CAD build for the part. Positions are in the model's coordinates, mm. A direction names the side the tool comes from. Round coordinates to 2 decimals unless told otherwise and drop trailing zeros. Loops run counter-clockwise (first coordinate to the right, second up) from the corner with the lowest first, then second, coordinate; pieces in that order, holes last. Notation, with made-up numbers: M -2.75,16.25 L 25.25,16.25 A10 cw 25.25,22.25 Z; hole C 11,59 d2. An arc over 180 degrees is marked long. One line per item, written item: value. Start each with the question number.
from build123d import *

# Parameters (mm, degrees)
AUFSATZ_LINEAR_AUSTRAGEN1_DEPTH = 8
DURCHGANGSLOCH_F_R_M5_D         = 5.5
DURCHGANGSLOCH_F_R_M4_D         = 4.5


with BuildPart() as part:
    # Skizze1 → Aufsatz-Linear austragen1 (new body)
    with BuildSketch(Plane.XY):
        with BuildLine():
            Line((4.5, -24.047375097), (-4.5, -24.047375097))
            ThreePointArc((-4.5, -24.047375097), (-6.621320344, -24.926054753), (-7.5, -27.047375097))
            Line((-7.5, -27.047375097), (-7.5, -28.047375097))
            Line((-7.5, -28.047375097), (-10.646349149, -28.047375097))
            ThreePointArc((-10.646349149, -28.047375097), (-15, -25.980762114), (-18.966564769, -23.243696368))
            Line((-18.966564769, -23.243696368), (-20.539739343, -20.518878077))
            Line((-20.539739343, -20.518878077), (-19.673713939, -20.018878077))
            ThreePointArc((-19.673713939, -20.018878077), (-18.27593646, -18.197259001), (-18.575637728, -15.920801865))
            Line((-18.575637728, -15.920801865), (-23.075637728, -8.126573231))
            ThreePointArc((-23.075637728, -8.126573231), (-24.897256804, -6.728795752), (-27.173713939, -7.02849702))
            Line((-27.173713939, -7.02849702), (-28.039739343, -7.52849702))
            Line((-28.039739343, -7.52849702), (-29.612913917, -4.803678728))
            ThreePointArc((-29.612913917, -4.803678728), (-28.775894551, 8.482210373), (-22.272727273, 20.097900881))
            ThreePointArc((-22.272727273, 20.097900881), (-21.699837667, 21.031080126), (-21.5, 22.107690969))
            Line((-21.5, 22.107690969), (-21.5, 38.107690969))
            Line((-21.5, 38.107690969), (-16.5, 40.107690969))
            Line((-16.5, 40.107690969), (-1.5, 40.107690969))
            Line((-1.5, 40.107690969), (-1.5, 8.9))
            Line((-1.5, 8.9), (-5.75, 8.9))
            ThreePointArc((-5.75, 8.9), (-10.871320344, 11.021320344), (-8.75, 5.9))
            Line((-8.75, 5.9), (-8.75, -5.459334644))
            ThreePointArc((-8.75, -5.459334644), (-8.536286844, -6.571362352), (-7.925596252, -7.524953425))
            ThreePointArc((-7.925596252, -7.524953425), (0, -10.928860874), (7.925596252, -7.524953425))
            ThreePointArc((7.925596252, -7.524953425), (8.536286844, -6.571362352), (8.75, -5.459334644))
            Line((8.75, -5.459334644), (8.75, 5.9))
            ThreePointArc((8.75, 5.9), (10.871320344, 11.021320344), (5.75, 8.9))
            Line((5.75, 8.9), (1.5, 8.9))
            Line((1.5, 8.9), (1.5, 40.107690969))
            Line((1.5, 40.107690969), (16.5, 40.107690969))
            Line((16.5, 40.107690969), (21.5, 38.107690969))
            Line((21.5, 38.107690969), (21.5, 22.107690969))
            ThreePointArc((21.5, 22.107690969), (21.699837667, 21.031080126), (22.272727273, 20.097900881))
            ThreePointArc((22.272727273, 20.097900881), (28.775894551, 8.482210373), (29.612913917, -4.803678728))
            Line((29.612913917, -4.803678728), (28.039739343, -7.52849702))
            Line((28.039739343, -7.52849702), (27.173713939, -7.02849702))
            ThreePointArc((27.173713939, -7.02849702), (24.897256804, -6.728795752), (23.075637728, -8.126573231))
            Line((23.075637728, -8.126573231), (18.575637728, -15.920801865))
            ThreePointArc((18.575637728, -15.920801865), (18.27593646, -18.197259001), (19.673713939, -20.018878077))
            Line((19.673713939, -20.018878077), (20.539739343, -20.518878077))
            Line((20.539739343, -20.518878077), (18.966564769, -23.243696368))
            ThreePointArc((18.966564769, -23.243696368), (15, -25.980762114), (10.646349149, -28.047375097))
            Line((10.646349149, -28.047375097), (7.5, -28.047375097))
            Line((7.5, -28.047375097), (7.5, -27.047375097))
            ThreePointArc((7.5, -27.047375097), (6.621320344, -24.926054753), (4.5, -24.047375097))
        make_face()
    extrude(amount=AUFSATZ_LINEAR_AUSTRAGEN1_DEPTH)

    # Durchgangsloch für M5 (through all)
    with Locations(Plane(origin=(21.5, 0, 0), x_dir=(0, 0, -1), z_dir=(1, 0, 0))):
        with Locations((-4, 31.107690969)):
            Hole(DURCHGANGSLOCH_F_R_M5_D / 2)

    # Durchgangsloch für M4 (through all)
    with Locations(Plane.XY.offset(8)):
        with Locations((-20, 0), (-10, 17.320508076), (10, 17.320508076), (20, 0), (10, -17.320508076), (-10, -17.320508076)):
            Hole(DURCHGANGSLOCH_F_R_M4_D / 2)


solid = part.part
(1) Slice it at B-B, the plane y = 0. List the corners of the cut face in (x, z), and give its area (3 significant figures).
(2) Slice it at D-D, the plane x = 25. List the corners of the cut face in (y, z).
(3) Which spindle directions (+Z, -Z, +X, -X, +Y, -Y) get a long thin tool onto all of the face, cutting with end or side? Do faces 1 (the flat face through (20.857, -11.969, 3.944)), 2 (the flat face through (1.5, 24, 4)), 3 (the flat face through (-8.75, 0, 4)), 4 (the cylindrical face through (-14.941, -26.014, 3.944)). Say none if no direction does.
(4) Mould opens along Y. For faces 5 (the flat face through (-1.5, 25, 4)), 6 (the cylindrical face through (-8.54, -6.56, 3.94)), 7 (the flat face through (-19.742, -21.9, 3.944)) say: pulls with the +Y half, pulls with the -Y half, needs draft (parallel to the pull), parting line crosses it, or undercut.
(5) Slice it at C-C, the plane z = 2.5. Count the separate pieces of the cut face and the enclosed holes in it, and give its area (3 significant figures).
(6) Probe L1, parallel to Y at x = 10, z = 3.75; L2, parallel to Y at x = -2.5, z = 3.25; L3, parallel to Y at x = -11.5, z = 3.5. List the from-to ranges inside material, lowest first.
(7) Flat gauge pins, fed straight in: P1, Ø2.5, axis at y = 3, z = 4.5, coming from the -X side; P2, Ø2, axis at x = -4, z = 4.5, coming from the -Y side; P3, Ø0.8, axis at y = -27.5, z = 3, coming from the -X side. Where does each tip first touch, or does it go through?
(8) Slice it at A-A, the plane y = 23.5. List the corners of the cut face in (x, z), and give its area (3 significant figures).
Check result:
1. outline: M -30,0 L -22.25,0 L -22.25,8 L -30,8 Z; M -17.75,0 L -8.75,0 L -8.75,8 L -17.75,8 Z; M 8.75,0 L 17.75,0 L 17.75,8 L 8.75,8 Z; M 22.25,0 L 30,0 L 30,8 L 22.25,8 Z
1. area: 268 mm^2
2. outline: M -6.7,0 L 16.58,0 L 16.58,8 L -6.7,8 Z
3. face 1: +Z, -Z, +X
3. face 2: +Z, -Z, +Y
3. face 3: +Z, -Z
3. face 4: +Z, -Z, -X, -Y
4. face 5: needs draft
4. face 6: undercut
4. face 7: pulls with the -Y half
5. separate pieces: 3
5. enclosed holes: 6
5. area: 2,380 mm^2
6. L1: y = -28.05 to -19.57, -15.07 to 6.17, 11.63 to 15.07, 19.57 to 28.37, 33.85 to 40.11
6. L2: y = -24.05 to -10.64, 8.9 to 28.46, 33.75 to 40.11
6. L3: y = -27.71 to -19, -15.64 to 7.7, 10.1 to 15.64, 19 to 28.4, 33.81 to 40.11
7. P1: stops at x = -29.95
7. P2: stops at y = -24.09
7. P3: stops at x = -12.87
8. outline: M -21.5,0 L -1.5,0 L -1.5,8 L -21.5,8 Z; M 1.5,0 L 21.5,0 L 21.5,8 L 1.5,8 Z
8. area: 320 mm^2
